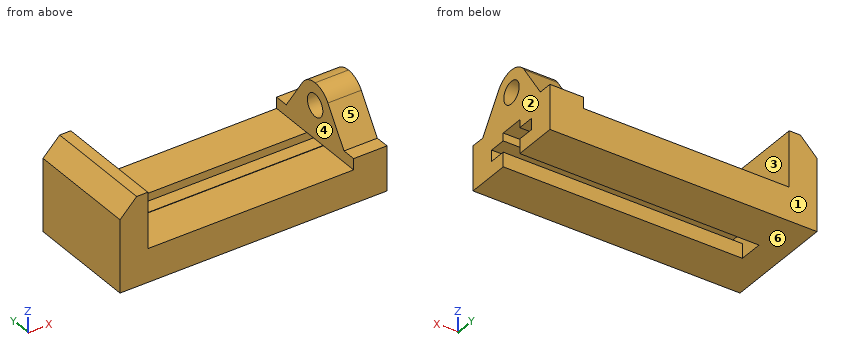
```python
from build123d import *

# Parameters (mm, degrees)
F0_W     = 304.8
F0_H     = 101.6
F1_DEPTH = 63.5
F2_W     = 234.95
F2_H     = 63.5
F3_DEPTH = 127.001
F4_SIZE2 = 19.05
F4_SIZE  = 19.05
F5_R     = 12.7
F6_DEPTH = 38.1
F8_DEPTH = 273.05


with BuildPart() as f1:
    # F0 (on Front) → F1 (new body, symmetric)
    with BuildSketch(Plane.XZ):
        with Locations((152.4, 50.8)):
            Rectangle(F0_W, F0_H)
    extrude(amount=F1_DEPTH, both=True)

    # F2 (on face) → F3 (cut, through all)
    with BuildSketch(Plane.XZ.offset(63.5)):
        with Locations((149.225, 69.85)):
            Rectangle(F2_W, F2_H)
    extrude(amount=-F3_DEPTH, mode=Mode.SUBTRACT)

    # F4
    f4_edges = [f1.edges().sort_by_distance(p)[0] for p in [
        (0, 0, 101.6),
    ]]
    chamfer(f4_edges, length=F4_SIZE, length2=F4_SIZE2)

    # F5 (on face) → F6 (cut)
    with BuildSketch(Plane.YZ.offset(304.8)):
        with BuildLine():
            Line((-63.5, 101.6), (-63.5, 50.8))
            Line((-63.5, 50.8), (-47.625, 50.8))
            Line((-47.625, 50.8), (-21.093426, 90.350173))
            ThreePointArc((-21.093426, 90.350173), (-11.952941, 98.611765), (0, 101.6))
            Line((0, 101.6), (-63.5, 101.6))
        make_face()
        with BuildLine():
            Line((63.5, 101.6), (0, 101.6))
            ThreePointArc((0, 101.6), (11.952941, 98.611765), (21.093426, 90.350173))
            Line((21.093426, 90.350173), (47.625, 50.8))
            Line((47.625, 50.8), (63.5, 50.8))
            Line((63.5, 50.8), (63.5, 101.6))
        make_face()
        with Locations((0, 76.2)):
            Circle(F5_R)
    extrude(amount=-F6_DEPTH, mode=Mode.SUBTRACT)

    # F7 (on face) → F8 (cut)
    with BuildSketch(Plane.YZ.offset(304.8)):
        Polygon((-13.675422, 0), (0, 0), (13.675422, 0), (13.675422, 16.51), (32.725422, 16.51), (32.725422, 29.21), (13.675422, 29.21), (13.675422, 38.1), (0, 38.1), (-13.675422, 38.1), (-13.675422, 29.21), (-32.725422, 29.21), (-32.725422, 16.51), (-13.675422, 16.51), align=None)
    extrude(amount=-F8_DEPTH, mode=Mode.SUBTRACT)


solid = f1.part
```
Geometry: final body of the model. Coordinates: model frame, mm. Face numbers are marked on the shaded views. A direction names the side the tool comes from. Round coordinates to 2 decimals unless told otherwise and drop trailing zeros. Order: outer loops, then holes, each group sorted by start corner. A loop starts at its lowest first (then second) coordinate and runs counter-clockwise, first axis right, second up. Notation, with made-up numbers: (82, 1) -> (110, 1) arc R34 ccw to (110, 35) -> close; hole circle Ø11 at (25.5, 74.5). An arc over 180 degrees is marked (long way). Use one line per item in the form item = value.
(1) Ray query, probe 1 along Z at (x, y) = (116, 21); probe 2 along Y at (x, z) = (272.5, 8); probe 3 along Z at (x, y) = (296, 0). Return the intervals inside material, ascending. Write a range as [from, to].
Results list:
probe_1 = [0, 16.51], [29.21, 38.1]
probe_2 = [-63.5, -13.68], [13.68, 63.5]
probe_3 = [38.1, 63.5], [88.9, 101.6]
(2) Section C-C on y = 4.5. Return loops of the section in (x, z), and give its area (3 significant figures).
Results list:
outline = (0, 0) -> (31.75, 0) -> (31.75, 101.6) -> (19.05, 101.6) -> (0, 82.55) -> close; (266.7, 38.1) -> (304.8, 38.1) -> (304.8, 64.32) -> (266.7, 64.32) -> close; (266.7, 88.08) -> (304.8, 88.08) -> (304.8, 101.2) -> (266.7, 101.2) -> close
area = 4,540 mm^2
(3) Section A-A on z = 44.5. Return loops of the section in (x, y).
Results list:
outline = (0, -63.5) -> (31.75, -63.5) -> (31.75, 63.5) -> (0, 63.5) -> close; (266.7, -63.5) -> (304.8, -63.5) -> (304.8, 63.5) -> (266.7, 63.5) -> close
(4) First-contact query: pin 1 Ø8 at (x, y) = (282, 4.5) entering from -Z; pin 2 Ø9.5 at (x, y) = (193.5, -23.5) entering from +Z; pin 3 Ø17.5 at (x, y) = (279.5, -56) entering from +Z; pin 4 Ø1 at (x, z) = (264.5, 74) entering from -Y. Flat tips, straight axial feed; report the tip coordinate or a pass-through.
Results list:
pin_1 = 38.1
pin_2 = 38.1
pin_3 = 51.36
pin_4 = through
(5) Access query for the marked faces 4, 5 and 6. Directions: +Z, -Z, +X, -X, +Y, -Y. A direction counts if a zero-diameter tool reaches every point of the face in a straight line with its end or side. Return the directions, or none.
Results list:
face_4 = +Z, +Y, -Y
face_5 = +Z, +X, -Y
face_6 = -Z, +X, -X, +Y, -Y
(6) Draft query along Y for the marked faces 1, 2 and 3. Return one class per face: pulls with the +Y half, pulls with the -Y half, needs draft (parallel to the pull), parting line crosses it, or undercut.
Results list:
face_1 = pulls with the +Y half
face_2 = needs draft
face_3 = undercut
(7) Section B-B on x = 186. Return loops of the section in (y, z), and give its area (3 significant figures).
Results list:
outline = (-63.5, 0) -> (-13.68, 0) -> (-13.68, 16.51) -> (-32.73, 16.51) -> (-32.73, 29.21) -> (-13.68, 29.21) -> (-13.68, 38.1) -> (-63.5, 38.1) -> close; (13.68, 0) -> (63.5, 0) -> (63.5, 38.1) -> (13.68, 38.1) -> (13.68, 29.21) -> (32.73, 29.21) -> (32.73, 16.51) -> (13.68, 16.51) -> close
area = 3,310 mm^2
(8) Section D-D on y = -38.5. Return loops of the section in (x, z), and give its area (3 significant figures).
Results list:
outline = (0, 0) -> (304.8, 0) -> (304.8, 64.4) -> (266.7, 64.4) -> (266.7, 38.1) -> (31.75, 38.1) -> (31.75, 101.6) -> (19.05, 101.6) -> (0, 82.55) -> close
area = 14,400 mm^2
